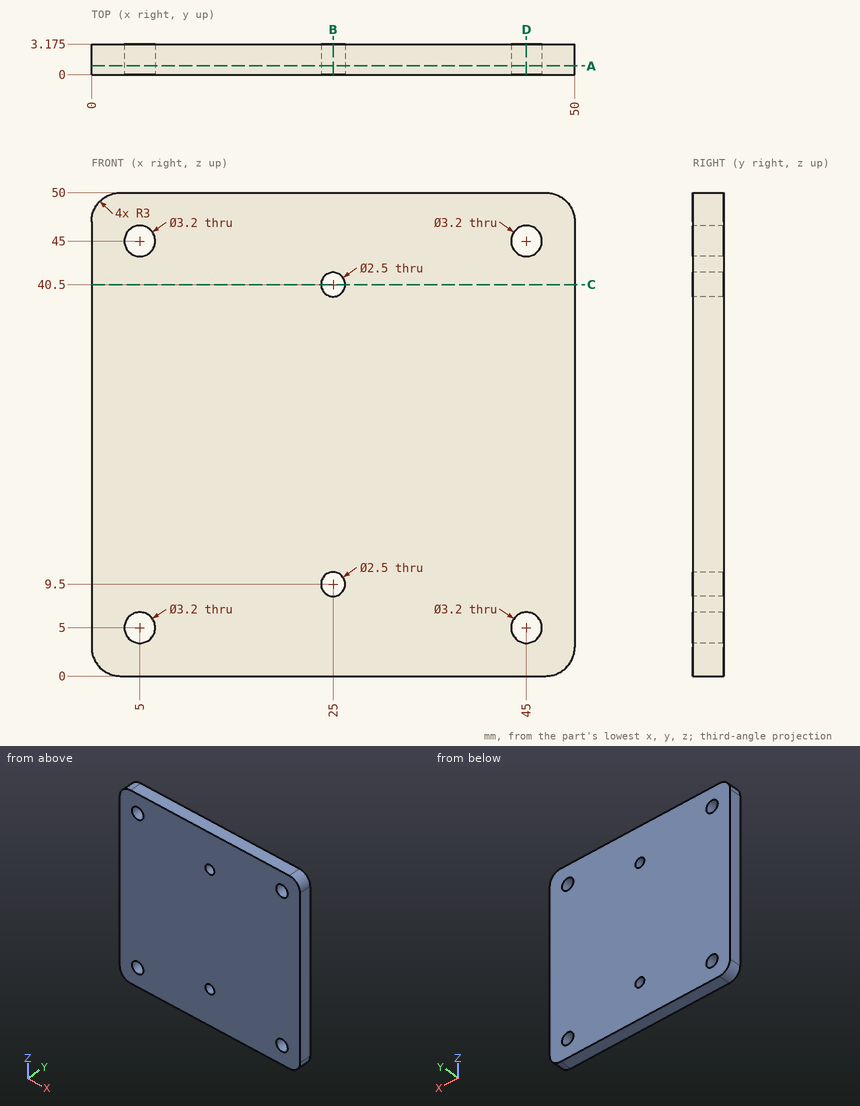
The figure shows three views and two pictorial views of one solid part (mm, origin at its lowest corner). Answer the questions. Give positions to 0.01 mm unless a question says otherwise; leave off trailing zeros. Order: outer loops, then holes, each group sorted by start corner. A loop starts at its lowest first (then second) coordinate and runs counter-clockwise, first axis right, second up. Notation, with made-up numbers: M 16,77 L 69,77 A10 cw 69,95 Z; hole C -17,61.25 d1. An arc over 180 degrees is marked long. Return JSON: item names as keys, results as strings.
Q1. Find section B-B, the plane x = 25. Write down the section's boundary in (y, z) (3 decimals), and give its area (3 significant figures).
Answer below:
{"outline": "M 0,0 L 3.175,0 L 3.175,8.25 L 0,8.25 Z; M 0,10.75 L 3.175,10.75 L 3.175,39.25 L 0,39.25 Z; M 0,41.75 L 3.175,41.75 L 3.175,50 L 0,50 Z", "area": "143 mm^2"}
Q2. Find section A-A, the plane y = 0.9. Write down the section's boundary in (x, z), and give its area (3 significant figures).
Answer below:
{"outline": "M 0,3 A3 ccw 3,0 L 47,0 A3 ccw 50,3 L 50,47 A3 ccw 47,50 L 3,50 A3 ccw 0,47 Z; hole C 5,5 d3.2; hole C 5,45 d3.2; hole C 25,9.5 d2.5; hole C 25,40.5 d2.5; hole C 45,5 d3.2; hole C 45,45 d3.2", "area": "2,450 mm^2"}
Q3. Find section C-C, the plane z = 40.5. Write down the section's boundary in (x, y) (3 decimals), and give its area (3 significant figures).
Answer below:
{"outline": "M 0,0 L 23.75,0 L 23.75,3.175 L 0,3.175 Z; M 26.25,0 L 50,0 L 50,3.175 L 26.25,3.175 Z", "area": "151 mm^2"}
Q4. Find the intervals of material crossed by line 1 along Z through (x, y) = (5, 0.75); line 2 along Z through (x, y) = (25, 0.7), in increasing order. Write a range as [from, to].
Answer below:
{"line 1": "z = [0, 3.4], [6.6, 43.4], [46.6, 50]", "line 2": "z = [0, 8.25], [10.75, 39.25], [41.75, 50]"}
Q5. Find section D-D, the plane x = 45. Write down the section's boundary in (y, z) (3 decimals).
Answer below:
{"outline": "M 0,0 L 3.175,0 L 3.175,3.4 L 0,3.4 Z; M 0,6.6 L 3.175,6.6 L 3.175,43.4 L 0,43.4 Z; M 0,46.6 L 3.175,46.6 L 3.175,50 L 0,50 Z"}
